Source: CAD feature listing. Evaluate the final solid. Frame: model axes, mm. A direction names the side the tool comes from. Coordinates: 2 decimals unless noted, no trailing zeros. Write each loop counter-clockwise with the first axis right and the second up, starting at its lowest first coordinate (ties: lowest second). Pieces come first, ordered by that corner, then holes. Notation, with made-up numbers: (27.5, 72) -> (73.5, 72) arc R18 ccw to (73.5, 82) -> close; hole circle Ø11 at (12.5, 34). An arc over 180 degrees is marked (long way). Write item = value, one per line.
from build123d import *

# Parameters (mm, degrees)
BOSS_EXTRUDE1_DEPTH = 19.05


with BuildPart() as part:
    # Sketch1 → Boss-Extrude1 (new body)
    with BuildSketch(Plane.XY):
        Polygon((6.3373, 3.658841861), (0, 7.317683722), (-6.3373, 3.658841861), (-6.3373, -3.658841861), (0, -7.317683722), (6.3373, -3.658841861), align=None)
        with BuildLine():
            ThreePointArc((3.9751, 0), (-2.435537513, -3.141588298), (-0.9906, 3.84969241))
            Line((-0.9906, 3.84969241), (-0.9906, 4.84029241))
            Line((-0.9906, 4.84029241), (0.9906, 4.84029241))
            Line((0.9906, 4.84029241), (0.9906, 3.84969241))
            ThreePointArc((0.9906, 3.84969241), (3.141588298, 2.435537513), (3.9751, 0))
        make_face(mode=Mode.SUBTRACT)
    extrude(amount=BOSS_EXTRUDE1_DEPTH)


solid = part.part
1) First-contact query: pin 1 Ø2 at (x, z) = (-3, 10.5) entering from +Y; pin 2 Ø1 at (x, z) = (3.5, 4) entering from +Y; pin 3 Ø5 at (x, z) = (0.5, 10.5) entering from -Y. Flat tips, straight axial feed; report the tip coordinate or a pass-through.
Answer block:
pin_1 = 6.16
pin_2 = 5.59
pin_3 = -7.32
2) Cut plane B-B, the plane y = -2.5. Output: boundary loops of the cut face in (x, z).
Answer block:
outline = (-6.34, 0) -> (-3.09, 0) -> (-3.09, 19.05) -> (-6.34, 19.05) -> close; (3.09, 0) -> (6.34, 0) -> (6.34, 19.05) -> (3.09, 19.05) -> close
3) Material intervals for probe 1 along X at (y, z) = (1.5, 4.25); probe 2 along Y at (x, z) = (-3.25, 9); probe 3 along X at (y, z) = (-3.25, 11.75), sorted ascending. Write a range as [from, to].
Answer block:
probe_1 = [-6.34, -3.68], [3.68, 6.34]
probe_2 = [-5.44, -2.29], [2.29, 5.44]
probe_3 = [-6.34, -2.29], [2.29, 6.34]
4) Cut plane C-C, the plane x = 5.5. Output: boundary loops of the cut face in (y, z), and give its area (3 significant figures).
Answer block:
outline = (-4.14, 0) -> (4.14, 0) -> (4.14, 19.05) -> (-4.14, 19.05) -> close
area = 158 mm2
5) Reachability of faces 5 (the flat face through (0, 4.84, 9)), 6 (the flat face through (6.337, 0, 9)) from +Z, -Z, +X, -X, +Y, -Y: full face, straight path, thin tool, end or side. Return the list, or none.
Answer block:
face_5 = +Z, -Z
face_6 = +Z, -Z, +X, +Y, -Y
6) Pull-direction query (Y, two-part tool) for faces 1 (the flat face through (-0.991, 4, 9)), 2 (the flat face through (-3.213, -5.463, 9.392)), 3 (the flat face through (-3, -3, 0)), 4 (the flat face through (0.991, 4, 9)); classes: +Y half, -Y half, draft (parallel to the pull), parting line (faces both ways), or undercut.
Answer block:
face_1 = undercut
face_2 = -Y half
face_3 = draft
face_4 = undercut
7) Cut plane A-A, the plane z = 2.75. Output: boundary loops of the cut face in (x, y).
Answer block:
outline = (-6.34, -3.66) -> (0, -7.32) -> (6.34, -3.66) -> (6.34, 3.66) -> (0, 7.32) -> (-6.34, 3.66) -> close; hole (-0.99, 3.85) arc R3.98 ccw (long way) to (0.99, 3.85) -> (0.99, 4.84) -> (-0.99, 4.84) -> close
8) Cut plane D-D, the plane y = -5.5. Output: boundary loops of the cut face in (x, z), and give its area (3 significant figures).
Answer block:
outline = (-3.15, 0) -> (3.15, 0) -> (3.15, 19.05) -> (-3.15, 19.05) -> close
area = 120 mm2
